from build123d import *

# Parameters (mm, degrees)
F0_W     = 50
F0_H     = 40.6
F1_DEPTH = 12.5
F3_DEPTH = 12.5
F4_W     = 50
F4_H     = 5.08
F5_DEPTH = 3.175
F6_R     = 1.27
F7_R     = 2.54


# Not quite as in the source:
# - a pattern or mirror of a feature is missing from the dataset's text; its kind, count and spacing are read off the source's solid
# - a feature names something its author has since deleted; it is built from what else it names


with BuildPart() as f1:
    # F0 (on Top) → F1 (new body)
    with BuildSketch(Plane.XY):
        Rectangle(F0_W, F0_H)
    extrude(amount=F1_DEPTH)

    # F2 (on face) → F3 (join, through all)
    with BuildSketch(Plane.XY.offset(12.5)):
        with BuildLine():
            Line((25, -2.875), (31.8612501666, -2.875))
            ThreePointArc((31.8612501666, -2.875), (42.05, 0), (31.8612501666, 2.875))
            Line((31.8612501666, 2.875), (25, 2.875))
            Line((25, 2.875), (25, 0))
            Line((25, 0), (25, -2.875))
        make_face()
    f3 = extrude(amount=-F3_DEPTH)

    # F3_copies: F3 across plane
    add(f3.mirror(Plane(origin=(0, 0, 0), x_dir=(0, 0, -1), z_dir=(-1, 0, 0))))

    # F4 (on face) → F5 (cut)
    with BuildSketch(Plane.XY.offset(12.5)):
        with Locations((0, 12.68)):
            Rectangle(F4_W, F4_H)
    f5 = extrude(amount=-F5_DEPTH, mode=Mode.SUBTRACT)

    # F5_copies: F5 across plane
    add(f5.mirror(Plane(origin=(0, 0, 0), x_dir=(0, 0, -1), z_dir=(0, -1, 0))), mode=Mode.SUBTRACT)

    # F6
    f6_edges = [f1.edges().sort_by_distance(p)[0] for p in [
        (0, 20.3, 12.5),
        (0, -20.3, 12.5),
        (0, 20.3, 0),
        (0, -20.3, 0),
    ]]
    fillet(f6_edges, radius=F6_R)

    # F7
    f7_edges = [f1.edges().sort_by_distance(p)[0] for p in [
        (0, 15.22, 12.5),
        (0, 10.14, 12.5),
        (0, -10.14, 12.5),
        (0, -15.22, 12.5),
    ]]
    fillet(f7_edges, radius=F7_R)


solid = f1.part
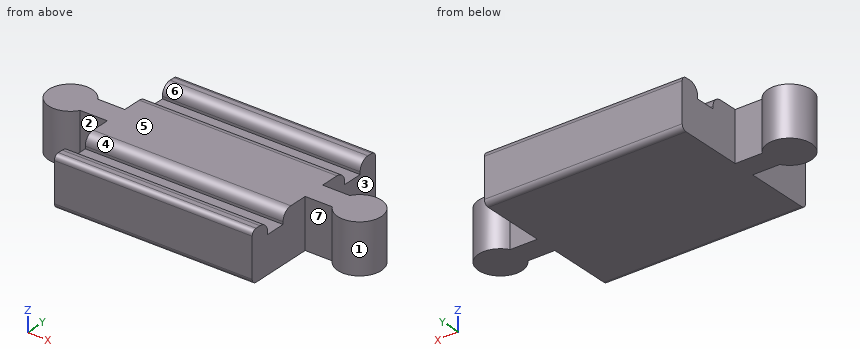
Model file for the job. Use its own axes, mm. Face numbers are marked on the shaded views. A direction names the side the tool comes from. Coordinates: 2 decimals unless noted, no trailing zeros. Order: outer loops, then holes, each group sorted by start corner. A loop starts at its lowest first (then second) coordinate and runs counter-clockwise, first axis right, second up. Notation, with made-up numbers: M 72.5,20.25 L 83.5,20.25 A21 ccw 83.5,58.25 Z; hole C 40.5,79 d7. An arc over 180 degrees is marked long. Return JSON: item names as keys, results as strings.
1. Pull direction Y, two halves, no side cores. Call the marked faces 4, 5, 6 and 7: +Y half, -Y half, draft (parallel to the pull), parting line (faces both ways), or undercut.
Ans:
{"face 4": "undercut", "face 5": "draft", "face 6": "undercut", "face 7": "-Y half"}
2. Drill centre lines: probe 1 along X at (y, z) = (4, 3.5); probe 2 along X at (y, z) = (-3.5, 9); probe 3 along Y at (x, z) = (1, 12). Where is each one in solid material? Low to high.
Ans:
{"probe 1": "-40.32 to -32.78, -25 to 25, 32.78 to 40.32", "probe 2": "-40.79 to -32.31, -25 to 25, 32.31 to 40.79", "probe 3": "-20.04 to -16.25, -9.11 to 9.11, 16.25 to 20.04"}
3. Saw through at D-D (x = -36.55). Give the cut face in (y, z).
Ans:
{"outline": "M -5.5,0 L 5.5,0 L 5.5,12.5 L -5.5,12.5 Z"}
4. Tool access for the marked faces 1, 2 and 3: list every direction of +Z, -Z, +X, -X, +Y, -Y with a clear straight run to the whole face (end or side of a thin tool).
Ans:
{"face 1": "+Z, -Z", "face 2": "+Z, -Z, -Y", "face 3": "+Z, -Z, +Y"}
5. Saw through at C-C (y = 4.5). Give the cut face in (x, z).
Ans:
{"outline": "M -39.71,0 L -33.39,0 L -33.39,12.5 L -39.71,12.5 Z; M -25,0 L 25,0 L 25,12.5 L -25,12.5 Z; M 33.39,0 L 39.71,0 L 39.71,12.5 L 33.39,12.5 Z"}
6. Flat gauge pins, fed straight in: pin 1 (5.5 mm diameter, centred on x = -4, y = 11.5, fed in from +Z); pin 2 (4 mm diameter, centred on y = -11, z = 8.5, fed in from +X); pin 3 (4 mm diameter, centred on x = 10, y = -12.5, fed in from +Z) (3 decimals). Where does each tip first touch, or does it go through?
Ans:
{"pin 1": "z = 12.22", "pin 2": "x = 25", "pin 3": "z = 9.325"}
7. Saw through at A-A (z = 4.25). Give the cut face in (x, y) (3 decimals), and give its area (3 significant figures).
Ans:
{"outline": "M -31.861,-2.875 L -25,-2.875 L -25,-20.3 L 25,-20.3 L 25,-2.875 L 31.861,-2.875 A5.5 ccw long 31.861,2.875 L 25,2.875 L 25,20.3 L -25,20.3 L -25,2.875 L -31.861,2.875 A5.5 ccw long Z", "area": "2,290 mm^2"}
8. Saw through at B-B (x = -21). Give the cut face in (y, z) (3 decimals).
Ans:
{"outline": "M -20.3,1.27 A1.27 ccw -19.03,0 L 19.03,0 A1.27 ccw 20.3,1.27 L 20.3,11.23 A1.27 ccw 19.03,12.5 L 17.76,12.5 A2.54 ccw 15.22,9.96 L 15.22,9.325 L 10.14,9.325 L 10.14,9.96 A2.54 ccw 7.6,12.5 L -7.6,12.5 A2.54 ccw -10.14,9.96 L -10.14,9.325 L -15.22,9.325 L -15.22,9.96 A2.54 ccw -17.76,12.5 L -19.03,12.5 A1.27 ccw -20.3,11.23 Z"}
